Job drawing, mm, ordinate dimensions from the low corner. One solid piece. A direction names the side the tool comes from. Round coordinates to 2 decimals unless told otherwise and drop trailing zeros. Loops run counter-clockwise (first coordinate to the right, second up) from the corner with the lowest first, then second, coordinate; pieces in that order, holes last.
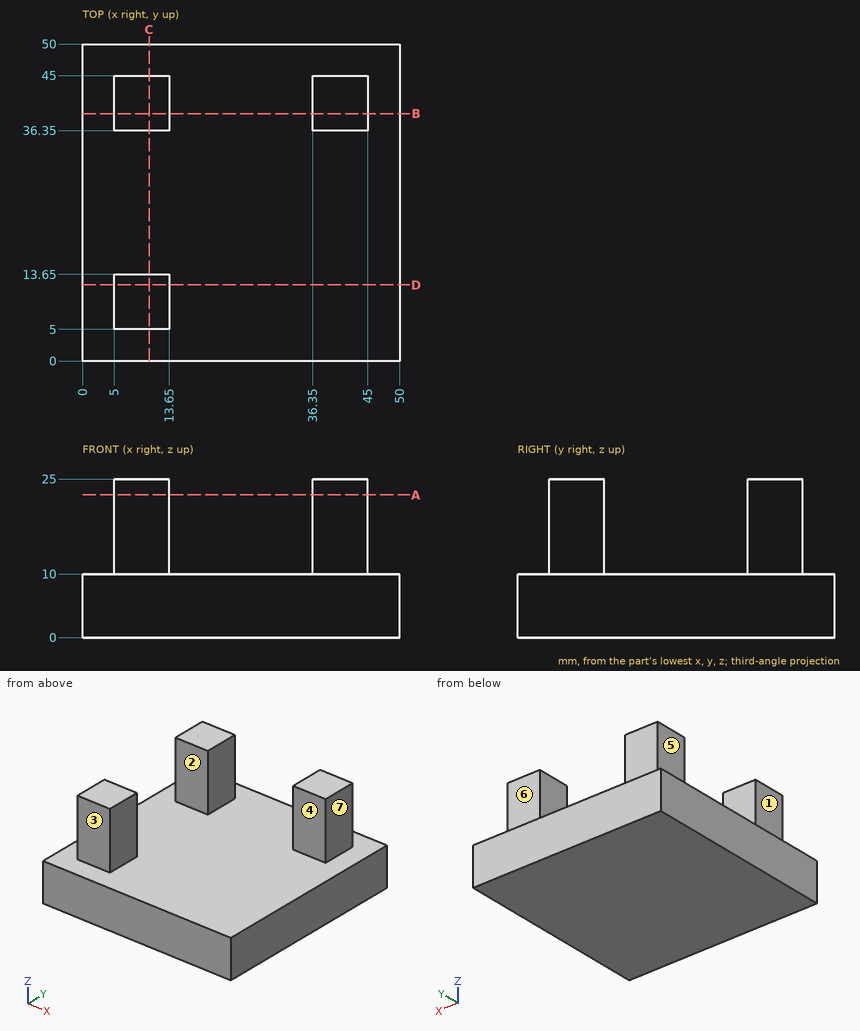
Item 1: Two-plate mould, pull along Y, no slides. Class the marked faces 1, 2 and 3: released by +Y, released by -Y, zero draft, split by the parting line, or undercut.
Answers follow:
face 1: zero draft
face 2: undercut
face 3: released by -Y
Item 2: 3-axis set-ups, long thin cutter, end or side, ignore diameter. For the marked faces 4, 5, 6 and 7: which of +Z, -Z, +X, -X, +Y, -Y reach the whole face in a straight line?
Answers follow:
face 4: +Z, +X, -X, -Y
face 5: +Z, -X, +Y, -Y
face 6: +Z, +X, -X, +Y
face 7: +Z, +X, +Y, -Y
Item 3: Cut at A-A, the plane z = 22.5. Give the cut face in (x, y).
Answers follow:
outline: (5, 5) - (13.65, 5) - (13.65, 13.65) - (5, 13.65) - close; (5, 36.35) - (13.65, 36.35) - (13.65, 45) - (5, 45) - close; (36.35, 36.35) - (45, 36.35) - (45, 45) - (36.35, 45) - close
Item 4: Cut at D-D, the plane y = 12. Give the cut face in (x, z).
Answers follow:
outline: (0, 0) - (50, 0) - (50, 10) - (13.65, 10) - (13.65, 25) - (5, 25) - (5, 10) - (0, 10) - close
Item 5: Flat gauge pins, fed straight in: P1, Ø2.5, axis at x = 8, z = 14.5, coming from the -Y side; P2, Ø2.5, axis at y = 40, z = 18, coming from the -X side; P3, Ø4.5, axis at x = 41.5, z = 14, coming from the +Y side. Where does each tip first touch, or does it go through?
Answers follow:
P1: stops at y = 5
P2: stops at x = 5
P3: stops at y = 45
Item 6: Cut at B-B, the plane y = 39. Give the cut face in (x, z), plus the area to 4 significant figures.
Answers follow:
outline: (0, 0) - (50, 0) - (50, 10) - (45, 10) - (45, 25) - (36.35, 25) - (36.35, 10) - (13.65, 10) - (13.65, 25) - (5, 25) - (5, 10) - (0, 10) - close
area: 759.5 mm2
Item 7: Probe line 1 (Y direction, x = 8.5, z = 21.5); line 2 (Z direction, x = 28, y = 45); line 3 (Y direction, x = 37, z = 12.25). List the from-to ranges inside material, lowest first.
Answers follow:
line 1: y = 5 to 13.65, 36.35 to 45
line 2: z = 0 to 10
line 3: y = 36.35 to 45
